from build123d import *

# Parameters (mm, degrees)
SKETCH1_W               = 101.6
SKETCH1_H               = 139.7
BOSS_EXTRUDE1_DEPTH     = 6.35
BOSS_EXTRUDE2_DEPTH     = 12.7
FILLET1_R               = 6.35
SKETCH3_R               = 3.175
CUT_EXTRUDE1_DEPTH      = 159.876949241
SKETCH4_R               = 6.7437
CUT_EXTRUDE2_DEPTH      = 3.175
SKETCH5_R               = 3.048
BOSS_EXTRUDE4_DEPTH     = 15.875
BOSS_EXTRUDE4_2_DEPTH   = 15.875
BOSS_EXTRUDE4_3_DEPTH   = 15.875
BOSS_EXTRUDE4_4_DEPTH   = 15.875
SKETCH6_R               = 6.6167
BOSS_EXTRUDE5_DEPTH     = 3.175
CUT_EXTRUDE3_DEPTH      = 2.54
CUT_EXTRUDE4_DEPTH      = 154.586010105
CUT_EXTRUDE4_DEPTH_BACK = 154.586010105
SKETCH8_R               = 3.5687
CHAMFER1_SIZE           = 1.27


with BuildPart() as part:
    # Sketch1 → Boss-Extrude1 (new body)
    with BuildSketch(Plane(origin=(0, 0, 0), x_dir=(1, 0, 0), z_dir=(0, 1, 0))):
        Rectangle(SKETCH1_W, SKETCH1_H)
        with BuildLine():
            Line((-40.0812, 28.5242), (-40.0812, 54.0258))
            ThreePointArc((-40.0812, 54.0258), (-34.925, 59.182), (-29.7688, 54.0258))
            Line((-29.7688, 54.0258), (-29.7688, 28.5242))
            ThreePointArc((-29.7688, 28.5242), (-34.925, 23.368), (-40.0812, 28.5242))
        make_face(mode=Mode.SUBTRACT)
        with BuildLine():
            Line((-40.0812, -54.0258), (-40.0812, -28.5242))
            ThreePointArc((-40.0812, -28.5242), (-34.925, -23.368), (-29.7688, -28.5242))
            Line((-29.7688, -28.5242), (-29.7688, -54.0258))
            ThreePointArc((-29.7688, -54.0258), (-34.925, -59.182), (-40.0812, -54.0258))
        make_face(mode=Mode.SUBTRACT)
        with BuildLine():
            Line((29.7688, -54.0258), (29.7688, -28.5242))
            ThreePointArc((29.7688, -28.5242), (34.925, -23.368), (40.0812, -28.5242))
            Line((40.0812, -28.5242), (40.0812, -54.0258))
            ThreePointArc((40.0812, -54.0258), (34.925, -59.182), (29.7688, -54.0258))
        make_face(mode=Mode.SUBTRACT)
        with BuildLine():
            Line((29.7688, 28.5242), (29.7688, 54.0258))
            ThreePointArc((29.7688, 54.0258), (34.925, 59.182), (40.0812, 54.0258))
            Line((40.0812, 54.0258), (40.0812, 28.5242))
            ThreePointArc((40.0812, 28.5242), (34.925, 23.368), (29.7688, 28.5242))
        make_face(mode=Mode.SUBTRACT)
    extrude(amount=-BOSS_EXTRUDE1_DEPTH)

    # Sketch2 → Boss-Extrude2 (add, symmetric)
    with BuildSketch(Plane(origin=(0, 0, 0), x_dir=(0, 0, -1), z_dir=(1, 0, 0))):
        with BuildLine():
            Line((63.6524, 0), (63.6524, 3.0226))
            ThreePointArc((63.6524, 3.0226), (62.725374501, 5.569581625), (60.378063539, 6.924802241))
            Line((60.378063539, 6.924802241), (19.2024, 14.185182671))
            Line((19.2024, 14.185182671), (19.2024, 127))
            Line((19.2024, 127), (12.8524, 127))
            Line((12.8524, 127), (12.8524, 0))
            Line((12.8524, 0), (63.6524, 0))
        make_face()
        with BuildLine():
            Line((-12.8524, 0), (-63.6524, 0))
            Line((-63.6524, 0), (-63.6524, 3.0226))
            ThreePointArc((-63.6524, 3.0226), (-62.725374501, 5.569581625), (-60.378063539, 6.924802241))
            Line((-60.378063539, 6.924802241), (-19.2024, 14.185182671))
            Line((-19.2024, 14.185182671), (-19.2024, 127))
            Line((-19.2024, 127), (-12.8524, 127))
            Line((-12.8524, 127), (-12.8524, 0))
        make_face()
    extrude(amount=BOSS_EXTRUDE2_DEPTH, both=True)

    # Fillet1
    fillet1_edges = [part.edges().sort_by_distance(p)[0] for p in [
        (0, 14.185182671, 19.2024),
        (0, 127, 19.2024),
        (0, 14.185182671, -19.2024),
        (0, 127, -19.2024),
    ]]
    fillet(fillet1_edges, radius=FILLET1_R - 0.0001)  # a hair under: the kernel refuses the full size

    # Sketch3 → Cut-Extrude1 (cut, through all)
    with BuildSketch(Plane.XZ.offset(6.35)):
        with Locations(Location((0, 50.546, 0), (0, 0, 270))):
            Circle(SKETCH3_R)
        with Locations(Location((0, 23.495, 0), (0, 0, 270))):
            Circle(SKETCH3_R)
        with Locations(Location((0, -23.495, 0), (0, 0, 270))):
            Circle(SKETCH3_R)
        with Locations(Location((0, -50.546, 0), (0, 0, 270))):
            Circle(SKETCH3_R)
    extrude(amount=-CUT_EXTRUDE1_DEPTH, mode=Mode.SUBTRACT)

    # Sketch4 → Cut-Extrude2 (cut)
    with BuildSketch(Plane.XZ.offset(6.35)):
        with Locations(Location((0, 50.546, 0), (0, 0, 270))):
            Circle(SKETCH4_R)
        with Locations(Location((0, 23.495, 0), (0, 0, 270))):
            Circle(SKETCH4_R)
        with Locations(Location((0, -23.495, 0), (0, 0, 270))):
            Circle(SKETCH4_R)
        with Locations(Location((0, -50.546, 0), (0, 0, 270))):
            Circle(SKETCH4_R)
    extrude(amount=-CUT_EXTRUDE2_DEPTH, mode=Mode.SUBTRACT)



with BuildPart() as body_2:
    # Sketch5 → Boss-Extrude4 (new body)
    with BuildSketch(Plane.XZ.offset(6.35)):
        with Locations(Location((0, 50.546, 0), (0, 0, 270))):
            Circle(SKETCH5_R)
    extrude(amount=-BOSS_EXTRUDE4_DEPTH)


with BuildPart() as body_3:
    # Sketch5 → Boss-Extrude4 2 (new body)
    with BuildSketch(Plane.XZ.offset(6.35)):
        with Locations(Location((0, 23.495, 0), (0, 0, 270))):
            Circle(SKETCH5_R)
    extrude(amount=-BOSS_EXTRUDE4_2_DEPTH)


with BuildPart() as body_4:
    # Sketch5 → Boss-Extrude4 3 (new body)
    with BuildSketch(Plane.XZ.offset(6.35)):
        with Locations(Location((0, -23.495, 0), (0, 0, 270))):
            Circle(SKETCH5_R)
    extrude(amount=-BOSS_EXTRUDE4_3_DEPTH)


with BuildPart() as body_5:
    # Sketch5 → Boss-Extrude4 4 (new body)
    with BuildSketch(Plane.XZ.offset(6.35)):
        with Locations(Location((0, -50.546, 0), (0, 0, 270))):
            Circle(SKETCH5_R)
    extrude(amount=-BOSS_EXTRUDE4_4_DEPTH)


with BuildPart() as part_1:
    add(part.part)

    add(body_2.part)  # Boss-Extrude5 merges body 2

    add(body_3.part)  # Boss-Extrude5 merges body 3

    add(body_4.part)  # Boss-Extrude5 merges body 4

    add(body_5.part)  # Boss-Extrude5 merges body 5
    # Sketch6 → Boss-Extrude5 (add)
    with BuildSketch(Plane.XZ.offset(6.35)):
        with Locations(Location((0, 23.495, 0), (0, 0, 270))):
            Circle(SKETCH6_R)
        with Locations(Location((0, 50.546, 0), (0, 0, 270))):
            Circle(SKETCH6_R)
        with Locations(Location((0, -23.495, 0), (0, 0, 270))):
            Circle(SKETCH6_R)
        with Locations(Location((0, -50.546, 0), (0, 0, 270))):
            Circle(SKETCH6_R)
    extrude(amount=-BOSS_EXTRUDE5_DEPTH)

    # Sketch7 → Cut-Extrude3 (cut)
    with BuildSketch(Plane.XZ.offset(6.35)):
        Polygon((0, 47.498), (2.639645431, 49.022), (2.639645431, 52.07), (0, 53.594), (-2.639645431, 52.07), (-2.639645431, 49.022), align=None)
        Polygon((0, 20.447), (2.639645431, 21.971), (2.639645431, 25.019), (0, 26.543), (-2.639645431, 25.019), (-2.639645431, 21.971), align=None)
        Polygon((0, -26.543), (2.639645431, -25.019), (2.639645431, -21.971), (0, -20.447), (-2.639645431, -21.971), (-2.639645431, -25.019), align=None)
        Polygon((0, -53.594), (2.639645431, -52.07), (2.639645431, -49.022), (0, -47.498), (-2.639645431, -49.022), (-2.639645431, -52.07), align=None)
    extrude(amount=-CUT_EXTRUDE3_DEPTH, mode=Mode.SUBTRACT)

    # Sketch8 → Cut-Extrude4 (cut, two sides: drawn at the far end of the back side and taken through both)
    with BuildSketch(Plane.XY.offset(-CUT_EXTRUDE4_DEPTH_BACK)):
        with Locations(Location((0, 69.85, 0), (0, 0, 270))):
            Circle(SKETCH8_R)
        with Locations(Location((0, 107.95, 0), (0, 0, 270))):
            Circle(SKETCH8_R)
    extrude(amount=CUT_EXTRUDE4_DEPTH + CUT_EXTRUDE4_DEPTH_BACK, mode=Mode.SUBTRACT)

    # Chamfer1
    chamfer1_edges = [part_1.edges().sort_by_distance(p)[0] for p in [
        (0, 9.525, 26.543),
        (0, 9.525, 53.594),
        (0, 9.525, -20.447),
        (0, 9.525, -47.498),
    ]]
    chamfer(chamfer1_edges, length=CHAMFER1_SIZE)


solid = part_1.part
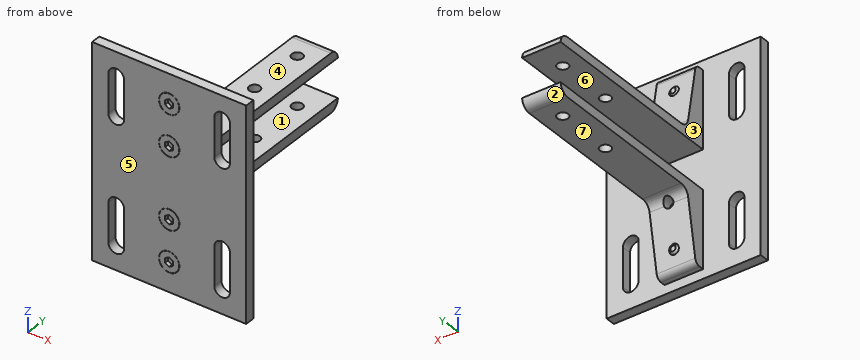
Check sheet for the modelled part. Datum: model origin and axes. Units: mm. Face numbers are marked on the shaded views. A direction names the side the tool comes from. Give positions to 0.01 mm unless a question says otherwise; leave off trailing zeros. Write each loop counter-clockwise with the first axis right and the second up, starting at its lowest first coordinate (ties: lowest second). Pieces come first, ordered by that corner, then holes. Notation, with made-up numbers: (30.5, 1) -> (82.5, 1) arc R16 ccw to (82.5, 32) -> close; hole circle Ø1 at (61, -29.75). An arc over 180 degrees is marked (long way). Write item = value, one per line.
Item 1: Sectioned sample at A-A on y = 39.5. Record the boundary of the cut face in (x, z), and give its area (3 significant figures).
Output:
outline = (-12.7, -19.2) -> (12.7, -19.2) -> (12.7, -12.85) -> (-12.7, -12.85) -> close; (-12.7, 12.85) -> (12.7, 12.85) -> (12.7, 19.2) -> (-12.7, 19.2) -> close
area = 323 mm^2
Item 2: Scan lines: probe 1 along Z at (x, y) = (5.5, 44); probe 2 along X at (y, z) = (69.85, 15); probe 3 along Y at (x, z) = (0, 15). Record each from-to range of solid material in increasing order. Write a range as from..to.
Output:
probe_1 = -19.2..-12.85, 12.85..19.2
probe_2 = -12.7..-3.57, 3.57..12.7
probe_3 = -6.35..66.28, 73.42..104.38, 111.52..126.63
Item 3: Release check for a two-part mould opening along Z. For the marked faces 5, 6 and 7 record: +Z half, -Z half, draft (parallel to the pull), parting line (faces both ways), or undercut.
Output:
face_5 = draft
face_6 = undercut
face_7 = -Z half
Item 4: Sectioned sample at C-C on z = -35.5. Record the boundary of the cut face in (x, y).
Output:
outline = (-50.8, -6.35) -> (-40.08, -6.35) -> (-40.08, 0) -> (-50.8, 0) -> close; (-29.77, -6.35) -> (29.77, -6.35) -> (29.77, 0) -> (12.7, 0) -> (12.7, 11.31) -> (-12.7, 11.31) -> (-12.7, 0) -> (-29.77, 0) -> close; (40.08, -6.35) -> (50.8, -6.35) -> (50.8, 0) -> (40.08, 0) -> close
Item 5: Sectioned sample at D-D on x = -35. Record the boundary of the cut face in (y, z), and give its area (3 significant figures).
Output:
outline = (-6.35, -69.85) -> (0, -69.85) -> (0, -59.18) -> (-6.35, -59.18) -> close; (-6.35, -23.37) -> (0, -23.37) -> (0, 23.37) -> (-6.35, 23.37) -> close; (-6.35, 59.18) -> (0, 59.18) -> (0, 69.85) -> (-6.35, 69.85) -> close
area = 432 mm^2
Item 6: Gauge pin test, flat ends, axial feed: pin 1 (1.9 mm diameter, centred on x = 1, z = 22, fed in from +Y) (3 decimals); pin 2 (4 mm diameter, centred on x = -40, z = 39, fed in from +Y); pin 3 (7.5 mm diameter, centred on x = 6, y = 54.5, fed in from +Z); pin 4 (4.5 mm diameter, centred on x = 0, y = 107.95, fed in from +Z). Record the tip position at first contact, or that the pin passes through.
Output:
pin_1 = 9.525
pin_2 = 0
pin_3 = 19.2
pin_4 = through
Item 7: Tool access check on the marked faces 1, 2, 3 and 4. Record the directions out of +Z, -Z, +X, -X, +Y, -Y that give a thin tool (end or side, any length) a straight path to the whole face; none if there is none.
Output:
face_1 = +X, -X, +Y
face_2 = -Z, +X, -X, +Y
face_3 = +Z, -Z, -X, +Y
face_4 = +Z, +X, -X, +Y
Item 8: Sectioned sample at B-B on y = 69.85. Record the boundary of the cut face in (x, z), and give its area (3 significant figures).
Output:
outline = (-12.7, -19.2) -> (-3.57, -19.2) -> (-3.57, -12.85) -> (-12.7, -12.85) -> close; (-12.7, 12.85) -> (-3.57, 12.85) -> (-3.57, 19.2) -> (-12.7, 19.2) -> close; (3.57, -19.2) -> (12.7, -19.2) -> (12.7, -12.85) -> (3.57, -12.85) -> close; (3.57, 12.85) -> (12.7, 12.85) -> (12.7, 19.2) -> (3.57, 19.2) -> close
area = 232 mm^2
